Autodesk Inventor part; units mm, degrees
ref_plane "YZ Plane" through (0, 0, 0) normal (1, 0, 0) x (0, 1, 0)
ref_plane "XZ Plane" through (0, 0, 0) normal (0, 1, 0) x (-1, 0, 0)
ref_plane "XY Plane" through (0, 0, 0) normal (0, 0, 1) x (1, 0, 0)
sketch "Sketch1" plane through (0, 0, 0) normal (0, 0, 1) x (1, 0, 0)
  line L0 (0, 0) -> (-18, 0)
  line L1 (-18, 0) -> (-18, 6)
  line L2 (-18, 6) -> (0, 6)
  line L3 (0, 6) -> (0, 0)
  dimension "d0" = 18
  dimension "d1" = 6
extrude "Extrusion1" add sketch "Sketch1" along normal blind 22
sketch "Sketch2" plane through (0, 0, 22) normal (0, 0, 1) x (1, 0, 0)
  line L0 (-18, 0) -> (0, 0)
  line L1 (0, 0) -> (0, 6)
  line L2 (0, 6) -> (-18, 6)
  line L3 (-18, 6) -> (-18, 0)
  circle A0 centre (-14.8, 3.2) radius 1.75
  circle A1 centre (-3.2, 3.2) radius 1.75
  dimension "d4" = 3.5
  dimension "d5" = 3.5
  dimension "d6" = 2.8
  dimension "d7" = 2.8
  dimension "d8" = 3.2
  dimension "d9" = 3.2
extrude "Extrusion2" cut sketch "Sketch2" against normal through all contours A0 | A1
sketch "Sketch3" plane through (0, 0, 0) normal (1, 0, 0) x (0, 0, -1)
  line L0 (0, 6) -> (0, 0)
  line L1 (0, 6) -> (-22, 6)
  line L2 (-22, 0) -> (-22, 6)
  line L3 (0, 0) -> (-22, 0)
  line L4 (0, 6) -> (-22, 6)
  line L5 (-22, 6) -> (-11.6, 6)
  line L6 (-11.6, 6) -> (-11.6, 21)
  line L7 (-11.6, 21) -> (-22, 21)
  line L8 (-22, 21) -> (-22, 6)
  dimension "d12" = 10.4
  dimension "d13" = 15
extrude "Extrusion3" add sketch "Sketch3" against normal up to surface (18 mm away) contours L1 L8 L7 L6
sketch "Sketch4" plane through (0, 6, 11.6) normal (0, 0, -1) x (-1, 0, 0)
  line L0 (18, 0) -> (18, 15)
  line L1 (0, 15) -> (18, 15)
  line L2 (0, 15) -> (0, 0)
  line L3 (18, 0) -> (0, 0)
  circle A0 centre (9, 8.7) radius 4.8
  point P0 (0, -6)
  dimension "d16" = 9.6
  dimension "d17" = 6.3
extrude "Extrusion4" cut sketch "Sketch4" against normal through all contours A0
sketch "Sketch5" plane through (-18, 0, 0) normal (-1, 0, 0) x (0, 0, 1)
  line L0 (22.0213, 0) -> (16.0213, 0)
  line L1 (16.0213, 0) -> (16.0213, 6)
  line L2 (16.0213, 6) -> (22.0213, 6)
  line L3 (22.0213, 6) -> (22.0213, 0)
  point P0 (0, 0)
  dimension "d20" = 6
  dimension "d21" = 6
extrude "Extrusion5" cut sketch "Sketch5" against normal blind 6
sketch "Sketch6" plane through (0, 0, 0) normal (1, 0, 0) x (0, 0, -1)
  line L0 (-22, 6) -> (-22, 0)
  line L1 (-16.0213, 6) -> (-22, 6)
  line L2 (-16.0213, 0) -> (-16.0213, 6)
  line L3 (-22, 0) -> (-16.0213, 0)
  point P0 (0, 0)
extrude "Extrusion6" cut sketch "Sketch6" against normal blind 6
sketch "Sketch7" plane through (0, 0, 0) normal (1, 0, 0) x (0, 0, -1)
  line L0 (-6.6, 12.2) -> (-11.6, 12.2)
  line L1 (-6.6, 17.2) -> (-11.6, 17.2)
  line L2 (-11.6, 21) -> (-11.6, 6)
  line L3 (-22, 6) -> (-22, 21)
  circle A0 centre (-16.8, 14.7) radius 1.4
  point P0 (0, 0)
  dimension "d26" = 2.8
  dimension "d27" = 5.2
  dimension "d28" = 2.5
extrude "Extrusion7" cut sketch "Sketch7" against normal blind 6
properties part number "00_micrometer_moun_xystage_china"
Geometry check sheet. Reference: the model listing, model coordinates, mm. A direction names the side the tool comes from. Coordinates: 2 decimals unless noted, no trailing zeros. Order: outer loops, then holes, each group sorted by start corner. A loop starts at its lowest first (then second) coordinate and runs counter-clockwise, first axis right, second up. Notation, with made-up numbers: (-18, -38.5) - (12, -38.5) arc R23 cw to (12, -4.5) - close; hole circle Ø3 at (-33.5, 8). An arc over 180 degrees is marked (long way). One line per item, written item: value.
(1) Sectioned sample at B-B (z = 12). Enter the section's corners in (x, y), and give its area (3 significant figures).
Data:
outline: (-18, 0) - (0, 0) - (0, 21) - (-18, 21) - close; hole circle Ø3.5 at (-14.8, 3.2); hole circle Ø9.6 at (-9, 14.7); hole circle Ø3.5 at (-3.2, 3.2)
area: 286 mm^2
(2) Sectioned sample at D-D (y = 3.2). Enter the section's corners in (x, z).
Data:
outline: (-18, 0) - (-16.55, 0) - (-16.55, 16.02) - (-18, 16.02) - close; (-13.05, 0) - (-4.95, 0) - (-4.95, 16.02) - (-6, 16.02) - (-6, 22) - (-12, 22) - (-12, 16.02) - (-13.05, 16.02) - close; (-1.45, 0) - (0, 0) - (0, 16.02) - (-1.45, 16.02) - close
(3) Release check for a two-part mould opening along Y. For faces 5 (the face through (-13.434, 12.862, 16.727)), 6 (the face through (-9, 0, 8)), 7 (the face through (-9, 3, 0)), 8 (the face through (-2.17, 13.85, 17.91)) record: +Y half, -Y half, draft (parallel to the pull), parting line (faces both ways), or undercut.
Data:
face 5: undercut
face 6: -Y half
face 7: draft
face 8: undercut
(4) Depth check by flat-ended pin: pin 1 Ø3.5 at (x, z) = (-7, 5.5) entering from +Y; pin 2 Ø1.8 at (y, z) = (1.5, 20) entering from -X; pin 3 Ø4 at (x, y) = (-3.2, 3.2) entering from +Z. Enter the tip coordinate at first touch or a pass-through.
Data:
pin 1: stops at y = 6
pin 2: stops at x = -12
pin 3: stops at z = 16.02
(5) Sectioned sample at A-A (x = -3.2). Enter the section's corners in (y, z).
Data:
outline: (0, 0) - (1.45, 0) - (1.45, 16.02) - (0, 16.02) - close; (4.95, 0) - (6, 0) - (6, 11.6) - (21, 11.6) - (21, 22) - (6, 22) - (6, 16.02) - (4.95, 16.02) - close; hole circle Ø2.8 at (14.7, 16.8)
(6) Access from +Z, -Z, +X, -X, +Y, -Y to the whole of each face (thin tool, end or side, straight path). Record for faces 1 (the face through (-3, 6, 19)), 2 (the face through (-9, 6, 6)), 3 (the face through (-16.4, 1.6, 16.021)), 4 (the face through (-13.99, 1.65, 8.12)).
Data:
face 1: +Z, +X, -Y
face 2: -Z, +X, -X, +Y
face 3: +Z, -X, -Y
face 4: +Z, -Z
(7) Thickness scan on probe 1 along Y at (x, z) = (-14.8, 10); probe 2 along Y at (x, z) = (-1.85, 16.8); probe 3 along Z at (x, y) = (-2.75, 14.7). Record the ranges inside material, lowest first. Write a range as from..to.
Data:
probe 1: y = 0..1.45, 4.95..6
probe 2: y = 6..13.3, 16.1..21
probe 3: z = 11.6..15.4, 18.2..22
(8) Sectioned sample at C-C (x = -14.8). Enter the section's corners in (y, z).
Data:
outline: (0, 0) - (1.45, 0) - (1.45, 16.02) - (0, 16.02) - close; (4.95, 0) - (6, 0) - (6, 11.6) - (21, 11.6) - (21, 22) - (6, 22) - (6, 16.02) - (4.95, 16.02) - close
